```python
from build123d import *

# Parameters (mm, degrees)
ESQUISSE1_W                 = 80
ESQUISSE1_H                 = 12.7
BOSS_EXTRU_1_DEPTH          = 12.7
TROU_TARAUD_M41_D           = 3.3
TROU_TARAUD_M41_CSINK_D     = 4.05
TROU_TARAUD_M41_CSINK_ANGLE = 90
ENL_V_START                 = -6.35
ENL_V_MAT_EXTRU_1_DEPTH     = 12.7


# Read off the part's stored shape, not the designer's step: Trou taraudé M51
with BuildPart() as part:
    # Esquisse1 → Boss.-Extru.1 (new body)
    with BuildSketch(Plane.XY):
        Rectangle(ESQUISSE1_W, ESQUISSE1_H)
    extrude(amount=BOSS_EXTRU_1_DEPTH)

    # Trou taraudé M41 (through all)
    with Locations(Plane.XY.offset(12.7)):
        with Locations((-35, 0), (-20, 0)):
            CounterSinkHole(TROU_TARAUD_M41_D / 2, TROU_TARAUD_M41_CSINK_D / 2, counter_sink_angle=TROU_TARAUD_M41_CSINK_ANGLE)

    # Esquisse4 → Enlèv. mat.-Extru.1 (cut)
    with BuildSketch(Plane(origin=(0, 0, 0), x_dir=(1, 0, 0), z_dir=(0, 1, 0)).offset(ENL_V_START)):
        with BuildLine():
            ThreePointArc((0, -3.704248689), (-7, -6.35), (0, -8.995751311))
            ThreePointArc((0, -8.995751311), (7, -6.35), (0, -3.704248689))
        make_face()
    extrude(amount=ENL_V_MAT_EXTRU_1_DEPTH, mode=Mode.SUBTRACT)

    # Trou taraudé M51 outline → Trou taraudé M51 (revolve, cut)
    with BuildSketch(Plane(origin=(35, 0, 0), x_dir=(1, 0, 0), z_dir=(0, -1, 0))):
        Polygon((0, 0), (2.1, 0), (2.1, 12.275), (2.525, 12.7), (0, 12.7), align=None)
    revolve(axis=Axis((35, 0, 0), (0, 0, 1)), mode=Mode.SUBTRACT)

    # Trou taraud_ M51 2 outline → Trou taraud_ M51 2 (revolve, cut)
    with BuildSketch(Plane(origin=(20, 0, 0), x_dir=(1, 0, 0), z_dir=(0, -1, 0))):
        Polygon((0, 0), (2.1, 0), (2.1, 12.275), (2.525, 12.7), (0, 12.7), align=None)
    revolve(axis=Axis((20, 0, 0), (0, 0, 1)), mode=Mode.SUBTRACT)


solid = part.part
```
For this review, take the finished solid that the model builds, in its own axes (mm). Round coordinates to 2 decimals unless told otherwise and drop trailing zeros. Write each loop counter-clockwise with the first axis right and the second up, starting at its lowest first coordinate (ties: lowest second). Pieces come first, ordered by that corner, then holes. Notation, with made-up numbers: (70, -12) -> (79, -12) arc R33 ccw to (79, 19) -> close; hole circle Ø10 at (78, -8.75). An arc over 180 degrees is marked (long way). One line per question, with ' | ' between items. Start each with the question number.
1) Add section D-D (y = 5). Write out the cut boundary in (x, z).
2) Add section C-C (x = 3). Write out the cut boundary in (y, z), and give its area (3 significant figures).
3) Add section B-B (x = -35). Write out the cut boundary in (y, z) (3 decimals).
4) For pin 1 Ø3 at (x, y) = (-20, 0) entering from +Z, flat-tipped, find the tip position at first contact; note if it passes through.
5) Wall thickness on line 1 along Z through (x, y) = (-3, -1.25); line 2 along X through (y, z) = (-1.75, 6.35); line 3 along X through (y, z) = (-0.5, 7.25): over which ranges is each line inside the solid? List them lowest first.
6) Add section A-A (z = 6.35). Write out the cut boundary in (x, y).
7) Mouldability with a two-part tool opening along Y and no side actions: class faces 1 (the cylindrical face through (32.9, 0.09, 6.22)), 2 (the flat face through (-1, 0, 12.7)), 3 (the flat face through (-1, -6.35, 10)) as +Y half, -Y half, draft (parallel to the pull), parting line (faces both ways), or undercut.
Reported:
1) outline: (-40, 0) -> (40, 0) -> (40, 12.7) -> (-40, 12.7) -> close; hole (0, 3.7) arc R4 ccw (long way) to (0, 9) arc R4 ccw (long way) to start
2) outline: (-6.35, 0) -> (6.35, 0) -> (6.35, 2.35) -> (-6.35, 2.35) -> close; (-6.35, 10.35) -> (6.35, 10.35) -> (6.35, 12.7) -> (-6.35, 12.7) -> close | area: 59.7 mm²
3) outline: (-6.35, 0) -> (-1.65, 0) -> (-1.65, 12.325) -> (-2.025, 12.7) -> (-6.35, 12.7) -> close; (1.65, 0) -> (6.35, 0) -> (6.35, 12.7) -> (2.025, 12.7) -> (1.65, 12.325) -> close
4) pin 1: passes through
5) line 1: z = 0 to 2.35, 10.35 to 12.7 | line 2: x = -40 to -7, 7 to 18.84, 21.16 to 33.84, 36.16 to 40 | line 3: x = -40 to -36.57, -33.43 to -21.57, -18.43 to -6.9, 6.9 to 17.96, 22.04 to 32.96, 37.04 to 40
6) outline: (-40, -6.35) -> (-7, -6.35) -> (-7, 6.35) -> (-40, 6.35) -> close; (7, -6.35) -> (40, -6.35) -> (40, 6.35) -> (7, 6.35) -> close; hole circle Ø3.3 at (-35, 0); hole circle Ø3.3 at (-20, 0); hole circle Ø4.2 at (20, 0); hole circle Ø4.2 at (35, 0)
7) face 1: undercut | face 2: draft | face 3: -Y half
